The model under review builds one solid part; all positions refer to its coordinate system, in mm. Coordinates: 2 decimals unless noted, no trailing zeros. Order: outer loops, then holes, each group sorted by start corner. A loop starts at its lowest first (then second) coordinate and runs counter-clockwise, first axis right, second up. Notation, with made-up numbers: (5, 39) -> (63, 39) arc R20 ccw to (63, 78) -> close; hole circle Ø3 at (-26.75, -10). An arc over 180 degrees is marked (long way). Put each result on its own line as item: value.
from build123d import *

# Parameters (mm, degrees)
SKETCH1_R           = 0.73533
SKETCH1_R_2         = 0.64516
BOSS_EXTRUDE1_DEPTH = 125
SKETCH2_W           = 1
SKETCH2_H           = 0.344184039
CUT_EXTRUDE1_DEPTH  = 10


with BuildPart() as part:
    # Sketch1 → Boss-Extrude1 (new body)
    with BuildSketch(Plane(origin=(0, 0, 0), x_dir=(1, 0, 0), z_dir=(0, 1, 0))):
        Circle(SKETCH1_R)
        Circle(SKETCH1_R_2, mode=Mode.SUBTRACT)
    extrude(amount=BOSS_EXTRUDE1_DEPTH)

    # Sketch2 → Cut-Extrude1 (cut)
    with BuildSketch(Plane.XZ):
        with Locations((0, -0.563237981)):
            Rectangle(SKETCH2_W, SKETCH2_H)
    extrude(amount=-CUT_EXTRUDE1_DEPTH, mode=Mode.SUBTRACT)


solid = part.part
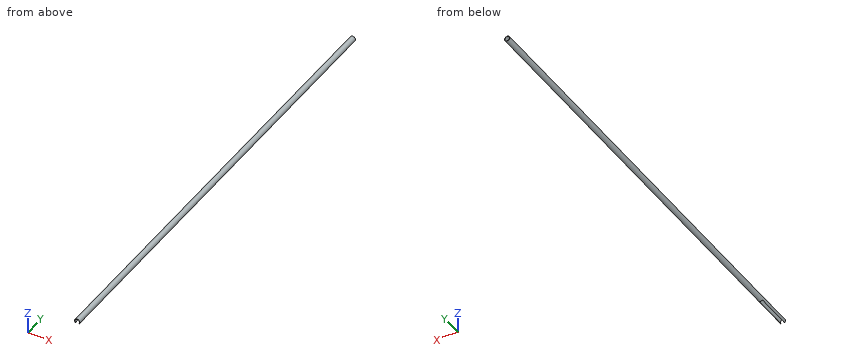
Item 1: Consider section A-A on z = 0. Write out the cut boundary in (x, y), and give its area (3 significant figures).
Answers below:
outline: (-0.74, 0) -> (-0.65, 0) -> (-0.65, 125) -> (-0.74, 125) -> close; (0.65, 0) -> (0.74, 0) -> (0.74, 125) -> (0.65, 125) -> close
area: 22.5 mm^2
Item 2: For pin 1 Ø0.8 at (x, z) = (0, 0) entering from +Y, flat-tipped, find the tip position at first contact; note if it passes through.
Answers below:
pin 1: through
Item 3: For line 1 (Z direction, x = 0.55, y = 18), list the stretches that pass through material, from the lowest coordinate up. Write a range as from..to.
Answers below:
line 1: -0.49..-0.34, 0.34..0.49
Item 4: Consider section B-B on x = 0. Write out the cut boundary in (y, z).
Answers below:
outline: (0, 0.65) -> (125, 0.65) -> (125, 0.74) -> (0, 0.74) -> close; (10, -0.74) -> (125, -0.74) -> (125, -0.65) -> (10, -0.65) -> close
Item 5: Consider section C-C on y = 25. Write out the cut boundary in (x, z), and give its area (3 significant figures).
Answers below:
outline: circle Ø1.47 at (0, 0); hole circle Ø1.29 at (0, 0)
area: 0.391 mm^2
